from build123d import *

# Parameters (mm, degrees)
BASE_EXTRUDE_DEPTH = 6.35
HOLE_CUTS_REACH    = 47.161
SKETCH2_R          = 1.905
TEETH_CUTS_REACH   = 47.161
TEETH_FILLET_R     = 0.381


with BuildPart() as part:
    # Sketch1 → Base Extrude (new body)
    with BuildSketch(Plane.XY):
        Polygon((0, 0), (6.35, 0), (11.43, 2.932939367), (33.02, 2.932939367), (38.1, 0), (44.45, 0), (44.45, 1.905), (38.1, 1.905), (33.02, 4.837939367), (11.43, 4.837939367), (6.35, 1.905), (0, 1.905), align=None)
    extrude(amount=BASE_EXTRUDE_DEPTH)

    # Sketch2 → Hole Cuts (cut, up to next)
    with BuildSketch(Plane(origin=(0, 4.837939367, 0), x_dir=(1, 0, 0), z_dir=(0, 1, 0)), mode=Mode.PRIVATE) as hole_cuts_sk1:
        with Locations(Location((41.275, -3.175, 0), (0, 0, 270))):
            Circle(SKETCH2_R)
    hole_cuts_tool1 = extrude(hole_cuts_sk1.sketch, amount=-HOLE_CUTS_REACH, mode=Mode.PRIVATE) & part.part
    # Sketch2 → Hole Cuts (cut, up to next)
    with BuildSketch(Plane(origin=(0, 4.837939367, 0), x_dir=(1, 0, 0), z_dir=(0, 1, 0)), mode=Mode.PRIVATE) as hole_cuts_sk2:
        with Locations(Location((3.175, -3.175, 0), (0, 0, 180))):
            Circle(SKETCH2_R)
    hole_cuts_tool2 = extrude(hole_cuts_sk2.sketch, amount=-HOLE_CUTS_REACH, mode=Mode.PRIVATE) & part.part
    add(hole_cuts_tool1.solids().sort_by_distance((41.275, 4.837939, 3.175))[0], mode=Mode.SUBTRACT)
    add(hole_cuts_tool2.solids().sort_by_distance((3.175, 4.837939, 3.175))[0], mode=Mode.SUBTRACT)

    # Sketch3 → Teeth Cuts (cut, up to next)
    with BuildSketch(Plane(origin=(0, 4.837939367, 0), x_dir=(1, 0, 0), z_dir=(0, 1, 0)), mode=Mode.PRIVATE) as teeth_cuts_sk1:
        Polygon((25.823333333, -6.35), (29.421666667, -6.35), (27.516666667, -2.54), align=None)
    teeth_cuts_tool1 = extrude(teeth_cuts_sk1.sketch, amount=-TEETH_CUTS_REACH, mode=Mode.PRIVATE) & part.part
    # Sketch3 → Teeth Cuts (cut, up to next)
    with BuildSketch(Plane(origin=(0, 4.837939367, 0), x_dir=(1, 0, 0), z_dir=(0, 1, 0)), mode=Mode.PRIVATE) as teeth_cuts_sk2:
        Polygon((29.421666667, -6.35), (33.02, -6.35), (31.115, -2.54), align=None)
    teeth_cuts_tool2 = extrude(teeth_cuts_sk2.sketch, amount=-TEETH_CUTS_REACH, mode=Mode.PRIVATE) & part.part
    # Sketch3 → Teeth Cuts (cut, up to next)
    with BuildSketch(Plane(origin=(0, 4.837939367, 0), x_dir=(1, 0, 0), z_dir=(0, 1, 0)), mode=Mode.PRIVATE) as teeth_cuts_sk3:
        Polygon((22.225, -6.35), (25.823333333, -6.35), (23.918333333, -2.54), align=None)
    teeth_cuts_tool3 = extrude(teeth_cuts_sk3.sketch, amount=-TEETH_CUTS_REACH, mode=Mode.PRIVATE) & part.part
    # Sketch3 → Teeth Cuts (cut, up to next)
    with BuildSketch(Plane(origin=(0, 4.837939367, 0), x_dir=(1, 0, 0), z_dir=(0, 1, 0)), mode=Mode.PRIVATE) as teeth_cuts_sk4:
        Polygon((18.626666667, -6.35), (22.225, -6.35), (20.32, -2.54), align=None)
    teeth_cuts_tool4 = extrude(teeth_cuts_sk4.sketch, amount=-TEETH_CUTS_REACH, mode=Mode.PRIVATE) & part.part
    # Sketch3 → Teeth Cuts (cut, up to next)
    with BuildSketch(Plane(origin=(0, 4.837939367, 0), x_dir=(1, 0, 0), z_dir=(0, 1, 0)), mode=Mode.PRIVATE) as teeth_cuts_sk5:
        Polygon((15.028333333, -6.35), (18.626666667, -6.35), (16.721666667, -2.54), align=None)
    teeth_cuts_tool5 = extrude(teeth_cuts_sk5.sketch, amount=-TEETH_CUTS_REACH, mode=Mode.PRIVATE) & part.part
    # Sketch3 → Teeth Cuts (cut, up to next)
    with BuildSketch(Plane(origin=(0, 4.837939367, 0), x_dir=(1, 0, 0), z_dir=(0, 1, 0)), mode=Mode.PRIVATE) as teeth_cuts_sk6:
        Polygon((11.43, -6.35), (15.028333333, -6.35), (13.123333333, -2.54), align=None)
    teeth_cuts_tool6 = extrude(teeth_cuts_sk6.sketch, amount=-TEETH_CUTS_REACH, mode=Mode.PRIVATE) & part.part
    add(teeth_cuts_tool1.solids().sort_by_distance((27.587222, 4.837939, 5.08))[0], mode=Mode.SUBTRACT)
    add(teeth_cuts_tool2.solids().sort_by_distance((31.185556, 4.837939, 5.08))[0], mode=Mode.SUBTRACT)
    add(teeth_cuts_tool3.solids().sort_by_distance((23.988889, 4.837939, 5.08))[0], mode=Mode.SUBTRACT)
    add(teeth_cuts_tool4.solids().sort_by_distance((20.390556, 4.837939, 5.08))[0], mode=Mode.SUBTRACT)
    add(teeth_cuts_tool5.solids().sort_by_distance((16.792222, 4.837939, 5.08))[0], mode=Mode.SUBTRACT)
    add(teeth_cuts_tool6.solids().sort_by_distance((13.193889, 4.837939, 5.08))[0], mode=Mode.SUBTRACT)

    # Teeth Fillet
    teeth_fillet_edges = [part.edges().sort_by_distance(p)[0] for p in [
        (29.421666667, 3.885439367, 6.35),
        (25.823333333, 3.885439367, 6.35),
        (18.626666667, 3.885439367, 6.35),
        (22.225, 3.885439367, 6.35),
        (15.028333333, 3.885439367, 6.35),
    ]]
    fillet(teeth_fillet_edges, radius=TEETH_FILLET_R)


solid = part.part
The model under review builds one solid part; all positions refer to its coordinate system, in mm. A direction names the side the tool comes from. Coordinates: 2 decimals unless noted, no trailing zeros. Write each loop counter-clockwise with the first axis right and the second up, starting at its lowest first coordinate (ties: lowest second). Pieces come first, ordered by that corner, then holes. Notation, with made-up numbers: M 47,61.25 L 85,61.25 A29 ccw 85,95.25 Z; hole C 84,38.25 d11. An arc over 180 degrees is marked long. Put each result on its own line as item: value.
1) Clearance check with flat-ended pins moving along their axes: pin 1 Ø3 at (x, z) = (43, 3.5) entering from +Y (3 decimals); pin 2 Ø3 at (x, z) = (3.175, 3.175) entering from -Y. State where each tip first meets the part, or that it passes through.
Computed:
pin 1: stops at y = 1.905
pin 2: passes through
2) Add section B-B on y = 2.3. Give the boundary of the cut face in (x, z).
Computed:
outline: M 7.03,0 L 10.33,0 L 10.33,6.35 L 7.03,6.35 Z; M 34.12,0 L 37.42,0 L 37.42,6.35 L 34.12,6.35 Z
3) Add section C-C on z = 0.5. Give the boundary of the cut face in (x, y) (3 decimals).
Computed:
outline: M 0,0 L 6.35,0 L 11.43,2.933 L 33.02,2.933 L 38.1,0 L 44.45,0 L 44.45,1.905 L 38.1,1.905 L 33.02,4.838 L 11.43,4.838 L 6.35,1.905 L 0,1.905 Z
4) For faces 4 (the flat face through (22, 2.933, 2)), 5 (the flat face through (19.65, 3.9, 4.05)), 6 (the flat face through (2, 1.905, 5)), 7 (the flat face through (6, 1, 6.35)), list the 3-axis set-ups (+Z, -Z, +X, -X, +Y, -Y) from which the entire face can be reached by the end or side of a thin tool; tool diameter is ignored.
Computed:
face 4: +Z, -Z, -Y
face 5: +Z, +Y, -Y
face 6: +Z, -Z, -X, +Y
face 7: +Z, +X, -X, +Y, -Y
5) Add section A-A on y = 0.65. Give the boundary of the cut face in (x, z) (3 decimals), then the cut area to 3 significant figures.
Computed:
outline: M 0,0 L 7.476,0 L 7.476,6.35 L 0,6.35 Z; M 36.974,0 L 44.45,0 L 44.45,6.35 L 36.974,6.35 Z; hole C 3.175,3.175 d3.81; hole C 41.275,3.175 d3.81
area: 72.1 mm2
6) Add section D-D on x = 21. Give the boundary of the cut face in (y, z).
Computed:
outline: M 2.93,0 L 4.84,0 L 4.84,3.9 L 2.93,3.9 Z
7) Draft analysis for pull direction Z (two halves, no side actions). For faces 1 (the flat face through (44.45, 1, 3)), 2 (the flat face through (17.5, 3.9, 4.1)), 3 (the cylindrical face through (43.164, 0.966, 2.927)), state which applies: released by +Z, released by -Z, zero draft, split by the parting line, or undercut.
Computed:
face 1: zero draft
face 2: released by +Z
face 3: undercut
8) Wall thickness on probe 1 along X at (y, z) = (1.75, 2.75); probe 2 along Y at (x, z) = (22, 3.25); probe 3 along Y at (x, z) = (38.5, 4) (3 decimals): over which ranges is each line inside the solid? List them lowest first. Write a range as [from, to].
Computed:
probe 1: x = [0, 1.32], [5.03, 9.38], [35.07, 39.42], [43.13, 44.45]
probe 2: y = [2.93, 4.84]
probe 3: y = [0, 1.905]
